The listing builds one solid part. Answer for the finished solid, in the listing's coordinates (mm). Face numbers are marked on the shaded views. Round coordinates to 2 decimals unless told otherwise and drop trailing zeros. Order: outer loops, then holes, each group sorted by start corner. A loop starts at its lowest first (then second) coordinate and runs counter-clockwise, first axis right, second up. Notation, with made-up numbers: (50, -32) - (60, -32) arc R7 ccw to (60, -22) - close; hole circle Ø7 at (-30.5, -24). An arc over 180 degrees is marked (long way). Write item = value, one per line.
from build123d import *

# Parameters (mm, degrees)
BOSS_EXTRUDE1_DEPTH = 12.7
CUT_EXTRUDE1_DEPTH  = 4.826
CUT_EXTRUDE2_DEPTH  = 4.826
SKETCH5_R           = 1.143
CUT_EXTRUDE3_DEPTH  = 296.565841373
SKETCH6_R           = 2.286
CUT_EXTRUDE4_DEPTH  = 294.076685716


with BuildPart() as part:
    # Sketch1 → Boss-Extrude1 (new body)
    with BuildSketch(Plane.XY):
        with BuildLine():
            Line((-0.759864647, 0.880311666), (-192.659480012, 223.198155833))
            ThreePointArc((-192.659480012, 223.198155833), (-192.85282615, 224.556676606), (-191.698096292, 225.298))
            Line((-191.698096292, 225.298), (-167.694919671, 225.298))
            ThreePointArc((-167.694919671, 225.298), (-166.637566458, 225.067459717), (-165.772152229, 224.417688334))
            Line((-165.772152229, 224.417688334), (26.127463136, 2.099844167))
            ThreePointArc((26.127463136, 2.099844167), (26.320809274, 0.741323394), (25.166079416, 0))
            Line((25.166079416, 0), (1.162902795, 0))
            ThreePointArc((1.162902795, 0), (0.105549582, 0.230540283), (-0.759864647, 0.880311666))
        make_face()
    extrude(amount=BOSS_EXTRUDE1_DEPTH)

    # Sketch3 → Cut-Extrude1 (cut)
    with BuildSketch(Plane.XY.offset(12.7)):
        Polygon((-183.376334539, 220.218), (2.32580559, 5.08), (16.844317663, 5.08), (-168.857822466, 220.218), align=None)
    extrude(amount=-CUT_EXTRUDE1_DEPTH, mode=Mode.SUBTRACT)

    # Sketch4 → Cut-Extrude2 (cut)
    with BuildSketch(Plane(origin=(0, 0, 0), x_dir=(-1, 0, 0), z_dir=(0, 0, -1))):
        Polygon((183.376334539, 220.218), (168.857822466, 220.218), (-16.844317663, 5.08), (-2.32580559, 5.08), align=None)
    extrude(amount=-CUT_EXTRUDE2_DEPTH, mode=Mode.SUBTRACT)

    # Sketch5 → Cut-Extrude3 (cut, through all)
    with BuildSketch(Plane.XZ.offset(-223.52)):
        with Locations((-176.948152229, 0)):
            Circle(SKETCH5_R)
        with Locations((-176.948152229, 12.7)):
            Circle(SKETCH5_R)
    extrude(amount=-CUT_EXTRUDE3_DEPTH, mode=Mode.SUBTRACT)

    # Sketch6 → Cut-Extrude4 (cut, through all)
    with BuildSketch(Plane(origin=(0, 5.08, 0), x_dir=(1, 0, 0), z_dir=(0, 1, 0))):
        with Locations((7.622135353, -12.7)):
            Circle(SKETCH6_R)
        with Locations((7.622135353, 0)):
            Circle(SKETCH6_R)
    extrude(amount=-CUT_EXTRUDE4_DEPTH, mode=Mode.SUBTRACT)


solid = part.part
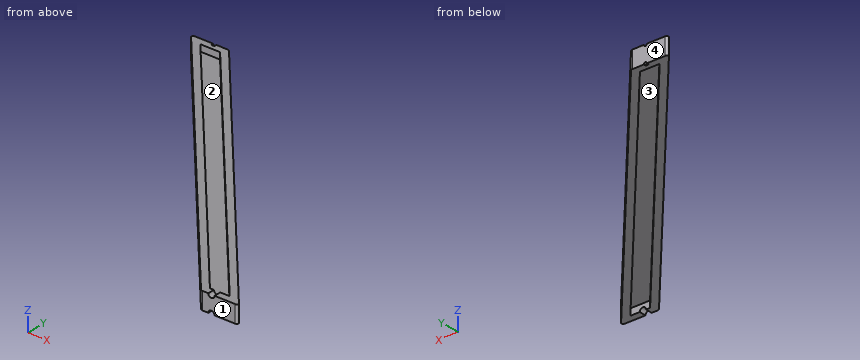
Q1. Section A-A on x = -25.5 is taken. Determine the outline of the cut face in (y, z), then the cut area to 3 significant figures.
Model answer:
outline = (29.54, 0) - (37.32, 0) - (37.32, 4.83) - (54.14, 4.83) - (54.14, 0) - (61.91, 0) - (61.91, 12.7) - (54.14, 12.7) - (54.14, 7.87) - (37.32, 7.87) - (37.32, 12.7) - (29.54, 12.7) - close
area = 249 mm^2
Q2. Section B-B on y = 39.5 is taken. Determine the outline of the cut face in (x, z), then the cut area to 3 significant figures.
Model answer:
outline = (-34.1, 0) - (-27.38, 0) - (-27.38, 4.83) - (-12.87, 4.83) - (-12.87, 0) - (-6.16, 0) - (-6.16, 12.7) - (-12.87, 12.7) - (-12.87, 7.87) - (-27.38, 7.87) - (-27.38, 12.7) - (-34.1, 12.7) - close
area = 215 mm^2
Q3. Find the intervals of material crossed by line 1 (X direction, y = 181, z = 8.75) (3 decimals); line 2 (Y direction, x = -106.5, z = 10.5); line 3 (X direction, y = 146, z = 8.25), in increasing order. Write a range as from..to.
Model answer:
line_1 = -156.235..-149.524, -135.006..-128.295
line_2 = 123.38..131.16, 147.98..155.75
line_3 = -126.02..-119.31, -104.79..-98.08
Q4. Determine the mould class of the marked faces 1, 2, 3 and 4 for opening direction Y: released by +Y, released by -Y, zero draft, split by the parting line, or undercut.
Model answer:
face_1 = released by -Y
face_2 = undercut
face_3 = undercut
face_4 = released by +Y
Q5. Flat-ended cylindrical pins translate along their axes: P1, Ø1, axis at y = 69.5, z = 9, coming from the -X side; P2, Ø5.5, axis at x = -178, z = 2.5, coming from the -Y side; P3, Ø6, axis at x = -3.5, z = 8.5, coming from the -Y side. Find the tip coordinate at first contact, or state that the pin passes through.
Model answer:
P1 = -60.42
P2 = 203.03
P3 = 0.62
